Answer from the drawing. Dimensions are ordinates in mm from the lowest x, y and z of the part. Coordinates: 2 decimals unless noted, no trailing zeros. Order: outer loops, then holes, each group sorted by start corner. A loop starts at its lowest first (then second) coordinate and runs counter-clockwise, first axis right, second up. Notation, with made-up numbers: M 65.5,-29 L 74.5,-29 A20 ccw 74.5,-19 Z; hole C 15.5,-16 d8. An arc over 180 degrees is marked long. One line per question, with ' | ' between items. Start each with the question number.
1) Given P1, Ø3, axis at x = 10, y = 8.45, coming from the -Z side, flat-ended and moving along its own axis, determine where the tip first touches the part or whether it passes through.
2) Find section D-D, the plane y = 7.5. Write down the section's boundary in (x, z) (1 decimal).
3) Find section A-A, the plane z = 8.75. Count the separate pieces of the cut face and the enclosed holes in it, plus the area to 3 significant figures.
4) Consider probe 1 along Y at (x, z) = (6, 7); probe 2 along Y at (x, z) = (11.75, 3.5); probe 3 along Y at (x, z) = (18.5, 11). Determine where each line is inside the solid, lowest interval first.
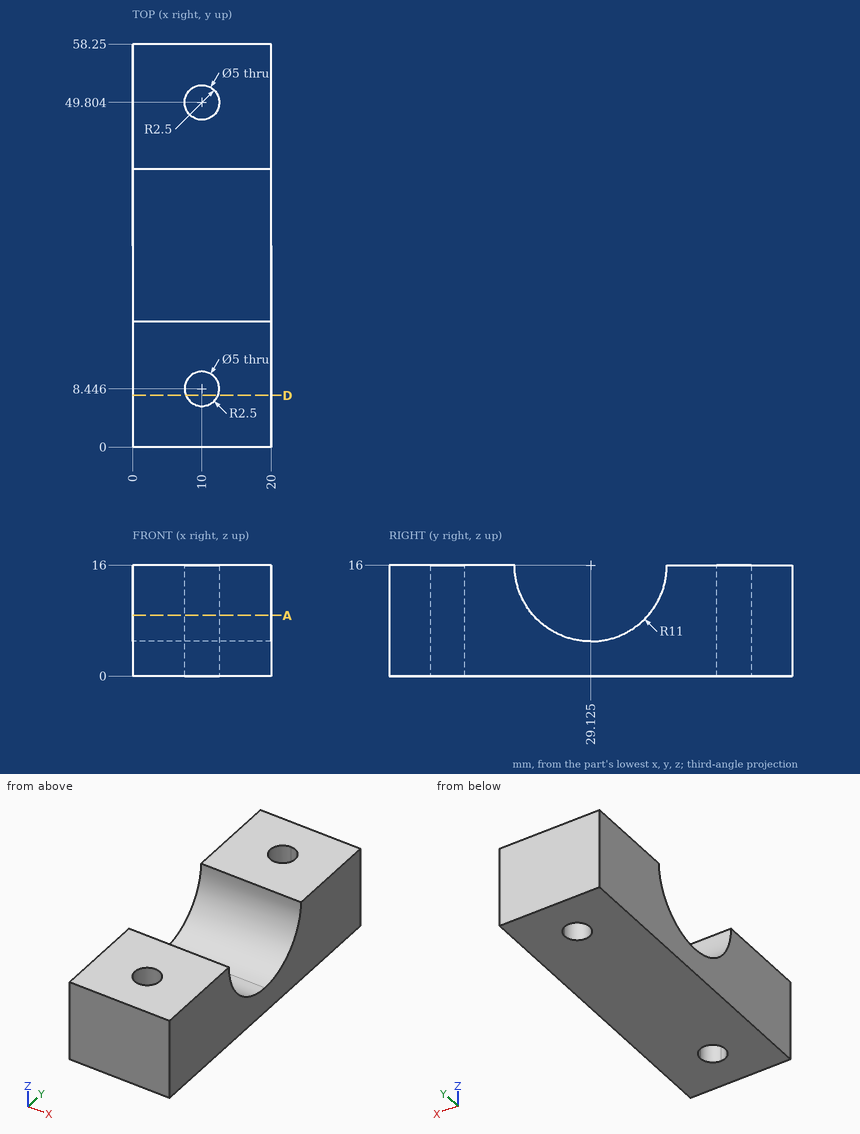
Report:
1) P1: passes through
2) outline: M 0,0 L 7.7,0 L 7.7,16 L 0,16 Z; M 12.3,0 L 20,0 L 20,16 L 12.3,16 Z
3) separate pieces: 2 | enclosed holes: 2 | area: 795 mm^2
4) probe 1: y = 0 to 22.8, 35.45 to 58.25 | probe 2: y = 0 to 6.66, 10.23 to 48.02, 51.59 to 58.25 | probe 3: y = 0 to 19.33, 38.92 to 58.25
